```python
from build123d import *

# Parameters (mm, degrees)
STRUCTURAL_MEMBER1_DEPTH = 50.8
SKETCH13_R               = 3
CUT_EXTRUDE1_DEPTH       = 45.745454998
SKETCH14_R               = 3
CUT_EXTRUDE2_DEPTH       = 45.745454998


with BuildPart() as part:
    # Sketch12 → Structural Member1 (new body)
    with BuildSketch(Plane.YZ.offset(-30.596662285)):
        with BuildLine():
            Line((0, 0), (0, 25))
            ThreePointArc((0, 25), (2.828427125, 23.828427125), (4, 21))
            Line((4, 21), (4, 7.5))
            ThreePointArc((4, 7.5), (5.025126266, 5.025126266), (7.5, 4))
            Line((7.5, 4), (21, 4))
            ThreePointArc((21, 4), (23.828427125, 2.828427125), (25, 0))
            Line((25, 0), (0, 0))
        make_face()
    extrude(amount=STRUCTURAL_MEMBER1_DEPTH)

    # Sketch13 → Cut-Extrude1 (cut, through all)
    with BuildSketch(Plane.XY.offset(4)):
        with Locations((-17.896662285, 12.7)):
            Circle(SKETCH13_R)
        with Locations((7.503337715, 12.7)):
            Circle(SKETCH13_R)
    extrude(amount=-CUT_EXTRUDE1_DEPTH, mode=Mode.SUBTRACT)

    # Sketch14 → Cut-Extrude2 (cut, through all)
    with BuildSketch(Plane(origin=(0, 4, 0), x_dir=(-1, 0, 0), z_dir=(0, 1, 0))):
        with Locations(Location((25.596662285, 15, 0), (0, 0, 90))):
            Circle(SKETCH14_R)
        with Locations(Location((0.196662285, 15, 0), (0, 0, 90))):
            Circle(SKETCH14_R)
    extrude(amount=-CUT_EXTRUDE2_DEPTH, mode=Mode.SUBTRACT)


solid = part.part
```
The model under review builds one solid part; all positions refer to its coordinate system, in mm. A direction names the side the tool comes from. Round coordinates to 2 decimals unless told otherwise and drop trailing zeros. Loops run counter-clockwise (first coordinate to the right, second up) from the corner with the lowest first, then second, coordinate; pieces in that order, holes last. Notation, with made-up numbers: (13, 82.5) - (68, 82.5) arc R22 cw to (68, 106.5) - close; hole circle Ø3 at (15.25, 5.5). An arc over 180 degrees is marked (long way). Use a Markdown table: item, result. Add a question column.
Q1. The part is to be moulded in two halves that separate along Y. For faces 3 (the face through (-20.894, 12.832, 2.028)), 4 (the face through (20.203, 4, 6)), 5 (the face through (-6, 0, 12)), say which applies: pulls with the +Y half, pulls with the -Y half, needs draft (parallel to the pull), parting line crosses it, or undercut.
Q2. Add section A-A (y = 12.7). State the section outline as (x, z) points.
Q3. For probe 1 along X at (y, z) = (2.95, 15); probe 2 along X at (y, z) = (3, 12.5); probe 3 along Y at (x, z) = (-17, 20), list the stretches that pass through material, from the lowest coordinate up.
Q4. Insertion check: pin 1 Ø5.5 at (x, z) = (-25.6, 15) entering from +Y; pin 2 Ø11 at (x, y) = (-14, 11.5) entering from +Z; pin 3 Ø11 at (x, z) = (-12.5, 13.5) entering from +Y; pin 4 Ø8 at (x, y) = (-17.9, 12.7) entering from +Z. Each pin has a flat end and moves straight along its axis. Give the tip position at first contact, or say it passes through.
Q5. Add section B-B (z = 15). State the section outline as (x, y) points, plus the area to 3 significant figures.
Q6. Add section D-D (x = 6.5). State the section outline as (y, z) points, plus the area to 3 significant figures.
Q7. Machinability: for faces 1 (the face through (-6, 4, 14)), 2 (the face through (-27.42, 2.03, 12.62)), which of the approach directions +Z, -Z, +X, -X, +Y, -Y give a long, thin tool a straight path to every point of the face, cutting with its end or side? Answer none if there is none.
Q8. Add section C-C (x = -5). State the section outline as (y, z) points, plus the area to 3 significant figures.
Worked answers:
| question | item | result |
|---|---|---|
| 1 | face 3 | undercut |
| 1 | face 4 | needs draft |
| 1 | face 5 | pulls with the -Y half |
| 2 | outline | (-30.6, 0) - (-20.9, 0) - (-20.9, 4) - (-30.6, 4) - close; (-14.9, 0) - (4.5, 0) - (4.5, 4) - (-14.9, 4) - close; (10.5, 0) - (20.2, 0) - (20.2, 4) - (10.5, 4) - close |
| 3 | probe 1 | -30.6 to -28.6, -22.6 to -3.2, 2.8 to 20.2 |
| 3 | probe 2 | -30.6 to -27.25, -23.94 to -1.85, 1.46 to 20.2 |
| 3 | probe 3 | 0 to 4 |
| 4 | pin 1 | through |
| 4 | pin 2 | z = 4.34 |
| 4 | pin 3 | y = 4 |
| 4 | pin 4 | z = 4 |
| 5 | outline | (-30.6, 0) - (-28.6, 0) - (-28.6, 4) - (-30.6, 4) - close; (-22.6, 0) - (-3.2, 0) - (-3.2, 4) - (-22.6, 4) - close; (2.8, 0) - (20.2, 0) - (20.2, 4) - (2.8, 4) - close |
| 5 | area | 155 mm² |
| 6 | outline | (0, 0) - (9.87, 0) - (9.87, 4) - (7.5, 4) arc R3.5 cw to (4, 7.5) - (4, 21) arc R4 ccw to (0, 25) - close; (15.53, 0) - (25, 0) arc R4 ccw to (21, 4) - (15.53, 4) - close |
| 6 | area | 157 mm² |
| 7 | face 1 | +Z, +X, -X, +Y |
| 7 | face 2 | +Y, -Y |
| 8 | outline | (0, 0) - (25, 0) arc R4 ccw to (21, 4) - (7.5, 4) arc R3.5 cw to (4, 7.5) - (4, 21) arc R4 ccw to (0, 25) - close |
| 8 | area | 180 mm² |
